from build123d import *

# Parameters (mm, degrees)
SKETCH1_R                = 8.562349171
BOSS_EXTRUDE1_DEPTH      = 20.32
BOSS_EXTRUDE2_START      = -2.833688097
SKETCH1_5_R              = 8.562349171
BOSS_EXTRUDE2_DEPTH      = 2.833688097
BOSS_EXTRUDE3_DEPTH      = 20.32
BOSS_EXTRUDE3_DEPTH_BACK = 2.833688097


with BuildPart() as part:
    # Sketch1 → Boss-Extrude1 (new body)
    with BuildSketch(Plane.YZ):
        with Locations(Location((0, 0, 0), (0, 0, 270))):
            Circle(SKETCH1_R)
    extrude(amount=BOSS_EXTRUDE1_DEPTH)

    # Sketch1<5> → Boss-Extrude2 (add)
    with BuildSketch(Plane.YZ.offset(BOSS_EXTRUDE2_START)):
        with Locations(Location((0, 0, 0), (0, 0, 180))):
            Circle(SKETCH1_5_R)
        with BuildLine():
            Line((8.562349171, 25.4), (-8.562349171, 25.4))
            Line((-8.562349171, 25.4), (-8.562349171, 0))
            ThreePointArc((-8.562349171, 0), (0, 8.562349171), (8.562349171, 0))
            Line((8.562349171, 0), (8.562349171, 25.4))
        make_face()
    extrude(amount=BOSS_EXTRUDE2_DEPTH)

    # Sketch1<6> → Boss-Extrude3 (add, two sides: drawn at the far end of the back side and taken through both)
    with BuildSketch(Plane.YZ.offset(-BOSS_EXTRUDE3_DEPTH_BACK)):
        Polygon((-33.554191153, 25.4), (-8.562349171, 25.4), (8.562349171, 25.4), (33.554191153, 25.4), (33.554191153, 83.9097483), (6.36016, 83.9097483), (6.36016, 79.644886138), (31.77032, 79.644886138), (31.77032, 41.557586138), (-31.77032, 41.557586138), (-31.77032, 79.644886138), (-6.36016, 79.644886138), (-6.36016, 83.9097483), (-33.554191153, 83.9097483), align=None)
    extrude(amount=BOSS_EXTRUDE3_DEPTH + BOSS_EXTRUDE3_DEPTH_BACK)


solid = part.part
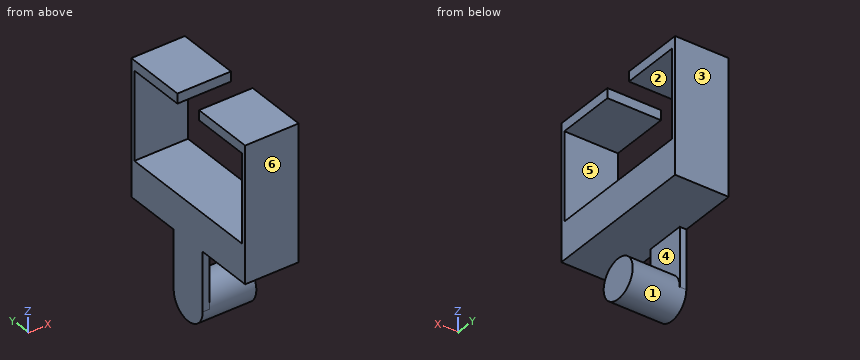
Can you work these out from the model? Positions are in its coordinate system, mm. Face numbers are marked on the shaded views. A direction names the side the tool comes from. Give positions to 0.01 mm unless a question says otherwise; leave off trailing zeros. Loops run counter-clockwise (first coordinate to the right, second up) from the corner with the lowest first, then second, coordinate; pieces in that order, holes last. Notation, with made-up numbers: M 58.5,44.25 L 94.5,44.25 A10 ccw 94.5,51.25 Z; hole C 58.5,78.25 d8. An arc over 180 degrees is marked long. One line per item, written item: value. Start each with the question number.
1) If we section it at D-D, the plane y = 0: Write out the boundary of the cut face in (x, z).
2) If we section it at C-C, the plane y = -27.5: Write out the boundary of the cut face in (x, z), and give its area (3 significant figures).
3) If I drill on line 1 (Z direction, x = 15.75, y = -23.5); line 2 (Y direction, x = 15.25, z = 66.5); line 3 (X direction, y = 3.5, z = 24), over which ranges is the centre line in solid material (lowest first)? Write a range as [from, to].
4) I'm going to push flat-ended pins straight in: pin 1 (7 mm diameter, centred on x = 8, y = 19.5, fed in from -Z); pin 2 (3 mm diameter, centred on x = -2, z = 14.5, fed in from +Y); pin 3 (1.4 mm diameter, centred on x = -2, z = 18.5, fed in from -Y). Where does each tip first touch, or does it pass through?
5) Thinking about a two-plate mould opening in Y: for the marked faces 4, 5 and 6, which applies, +Y half, -Y half, draft (parallel to the pull), parting line (faces both ways), or undercut?
6) On a 3-axis mill with a long thin cutter (end or side, diameter ignored), from which of +Z, -Z, +X, -X, +Y, -Y can I reach the whole of each face in a straight line? I mean the marked faces 1, 2 and 3. Say none if no direction works.
7) If we section it at A-A, the plane x = 2.25: Write out the boundary of the cut face in (y, z), and give its area (3 significant figures).
8) If we section it at B-B, the plane z = 73: Write out the boundary of the cut face in (x, y).
Completed:
1. outline: M -2.83,-8.56 L 20.32,-8.56 L 20.32,8.56 L 0,8.56 L 0,25.4 L 20.32,25.4 L 20.32,41.56 L -2.83,41.56 Z
2. outline: M -2.83,25.4 L 20.32,25.4 L 20.32,41.56 L -2.83,41.56 Z; M -2.83,79.64 L 20.32,79.64 L 20.32,83.91 L -2.83,83.91 Z
2. area: 473 mm^2
3. line 1: z = [25.4, 41.56], [79.64, 83.91]
3. line 2: y = [-33.55, -31.77], [31.77, 33.55]
3. line 3: x = [-2.83, 0]
4. pin 1: stops at z = 25.4
4. pin 2: stops at y = 8.56
4. pin 3: stops at y = -8.56
5. face 4: draft
5. face 5: undercut
5. face 6: -Y half
6. face 1: +X
6. face 2: +X, -X
6. face 3: +Z, -Z, +X, -X, +Y
7. outline: M -33.55,25.4 L 33.55,25.4 L 33.55,83.91 L 6.36,83.91 L 6.36,79.64 L 31.77,79.64 L 31.77,41.56 L -31.77,41.56 L -31.77,79.64 L -6.36,79.64 L -6.36,83.91 L -33.55,83.91 Z; C 0,0 d17.12
7. area: 1,680 mm^2
8. outline: M -2.83,-33.55 L 20.32,-33.55 L 20.32,-31.77 L -2.83,-31.77 Z; M -2.83,31.77 L 20.32,31.77 L 20.32,33.55 L -2.83,33.55 Z
